Here's how the part is built. I have some questions about the finished solid (model axes, mm). Face numbers are marked on the shaded views. A direction names the side the tool comes from. Coordinates: 2 decimals unless noted, no trailing zeros. Write each loop counter-clockwise with the first axis right and the second up, starting at its lowest first coordinate (ties: lowest second). Pieces come first, ordered by that corner, then holes. Notation, with made-up numbers: (60, 30.5) -> (94, 30.5) arc R31 ccw to (94, 62.5) -> close; hole circle Ø6 at (68.25, 18.5). An arc over 180 degrees is marked (long way). Put each result on its own line as item: value.
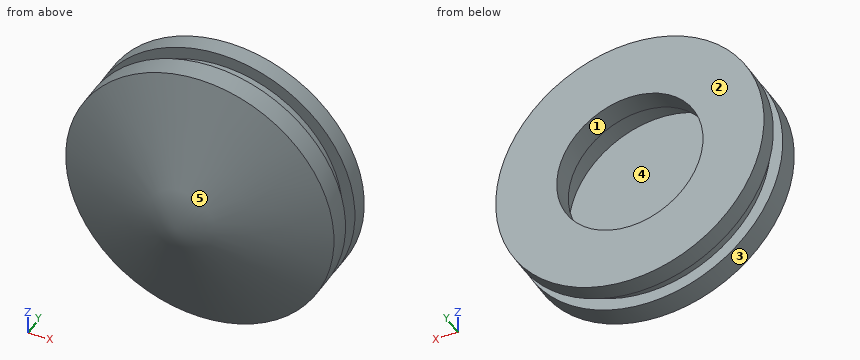
```python
from build123d import *


with BuildPart() as part:
    # Esquisse1 → Révolution1 (revolve)
    with BuildSketch(Plane.XY, mode=Mode.PRIVATE) as r_volution1_sk:
        Polygon((0, 0), (0, 8.853672577), (-11, 8.853672577), (-11, 7.353672577), (-10, 7.353672577), (-10, 5.853672577), (-11, 5.853672577), (-11, 4.003672577), align=None)
    revolve(r_volution1_sk.sketch.rotate(Axis((0, 0, 0), (0, 1, 0)), 270), axis=Axis((0, 0, 0), (0, 1, 0)))

    # Esquisse3 → Enlèvement de matière-Révolution1 (revolve, cut)
    with BuildSketch(Plane.XY, mode=Mode.PRIVATE) as enl_vement_de_mati_re_r_volution1_sk:
        Polygon((-6, 10), (-6, 7), (-7.5, 7), (-7.5, 4.003672577), (0, 4.003672577), (0, 10), align=None)
    revolve(enl_vement_de_mati_re_r_volution1_sk.sketch.rotate(Axis((0, 0, 0), (0, 1, 0)), 270), axis=Axis((0, 0, 0), (0, 1, 0)), mode=Mode.SUBTRACT)


solid = part.part
```
Item 1: Which directions (+Z, -Z, +X, -X, +Y, -Y) give clear straight access to the entire face, cutting with the end or side of a thin tool? Please do the marked faces 1 and 2.
Output:
face 1: +Y
face 2: +Z, -Z, +X, -X, +Y
Item 2: Please list where these lines run through material, in increasing order: line 1 along X through (y, z) = (8.5, 0); line 2 along X through (y, z) = (6.1, 0); line 3 along Y through (x, z) = (-7.75, -6.5). Write a range as from..to.
Output:
line 1: x = -11..-6, 6..11
line 2: x = -10..-7.5, 7.5..10
line 3: y = 3.68..5.85, 7.35..8.85
Item 3: If we mould it in two halves opening along Y, with no side actions, what happens to the marked faces 3, 4 and 5? For each: released by +Y, released by -Y, zero draft, split by the parting line, or undercut.
Output:
face 3: zero draft
face 4: undercut
face 5: released by -Y
Item 4: Imagine slicing it at B-B on y = 2.5. Write out the boundary of the cut face in (x, z).
Output:
outline: circle Ø13.74 at (0, 0)
Item 5: Imagine slicing it at A-A on y = 1. Write out the boundary of the cut face in (x, z), then the cut area to 3 significant figures.
Output:
outline: circle Ø5.49 at (0, 0)
area: 23.7 mm²
Item 6: For P1, Ø2, axis at y = 3.5, z = 2.5, coming from the +X side; P2, Ø12, axis at x = -2.5, z = 6.5, coming from the -Y side; P3, Ø9, axis at x = 0, z = 0, coming from the +Y side, each with a flat end and sliding along its axis, tell me the tip position at first contact or that it passes through.
Output:
P1: stops at x = 10.88
P2: stops at y = 0.35
P3: stops at y = 4
